Verification items for the finished model (mm, model axes). A direction names the side the tool comes from. Give positions to 0.01 mm unless a question says otherwise; leave off trailing zeros. Order: outer loops, then holes, each group sorted by start corner. A loop starts at its lowest first (then second) coordinate and runs counter-clockwise, first axis right, second up.
from build123d import *

# Parameters (mm, degrees)
BOSS_EXTRUDE1_DEPTH = 6.353
CUT_EXTRUDE1_REACH  = 30.604
SKETCH2_R           = 1.75
SKETCH3_R           = 32.5
CUT_EXTRUDE2_DEPTH  = 9.675
FILLET1_R           = 2.5
CHAMFER1_SIZE       = 10
CHAMFER1_SIZE2      = 1.763269807
CHAMFER2_SIZE       = 10
CHAMFER2_SIZE2      = 1.763269807


with BuildPart() as part:
    # Sketch1 → Boss-Extrude1 (new body)
    with BuildSketch(Plane(origin=(0, 0, 0), x_dir=(0, 0, -1), z_dir=(1, 0, 0))):
        Polygon((0, 19.4375), (-20, 19.4375), (-20, -19.4375), (20, -19.4375), (20, -16.2625), (0, -16.2625), (0, -9.7625), (20, -9.7625), (20, 5.0375), (0, 5.0375), (0, 11.5375), align=None)
    extrude(amount=BOSS_EXTRUDE1_DEPTH)

    # Sketch2 → Cut-Extrude1 (cut, up to next)
    with BuildSketch(Plane(origin=(6.353, 0, 0), x_dir=(0, 0, -1), z_dir=(1, 0, 0)), mode=Mode.PRIVATE) as cut_extrude1_sk1:
        with BuildLine():
            ThreePointArc((-16.45, 5.8875), (-14.7, 7.6375), (-12.95, 5.8875))
            ThreePointArc((-12.95, 5.8875), (-12.455196051, 8.612317472), (-11.033966385, 10.989199346))
            ThreePointArc((-11.033966385, 10.989199346), (-11.199317007, 13.458543221), (-13.668660882, 13.293192599))
            ThreePointArc((-13.668660882, 13.293192599), (-15.731736204, 9.842880202), (-16.45, 5.8875))
        make_face()
    cut_extrude1_tool1 = extrude(cut_extrude1_sk1.sketch, amount=-CUT_EXTRUDE1_REACH, mode=Mode.PRIVATE) & part.part
    # Sketch2 → Cut-Extrude1 (cut, up to next)
    with BuildSketch(Plane(origin=(6.353, 0, 0), x_dir=(0, 0, -1), z_dir=(1, 0, 0)), mode=Mode.PRIVATE) as cut_extrude1_sk2:
        with Locations((-14.7, 5.8875)):
            Circle(SKETCH2_R)
    cut_extrude1_tool2 = extrude(cut_extrude1_sk2.sketch, amount=-CUT_EXTRUDE1_REACH, mode=Mode.PRIVATE) & part.part
    # Sketch2 → Cut-Extrude1 (cut, up to next)
    with BuildSketch(Plane(origin=(6.353, 0, 0), x_dir=(0, 0, -1), z_dir=(1, 0, 0)), mode=Mode.PRIVATE) as cut_extrude1_sk3:
        with Locations((-5.2, 5.8875)):
            Circle(SKETCH2_R)
    cut_extrude1_tool3 = extrude(cut_extrude1_sk3.sketch, amount=-CUT_EXTRUDE1_REACH, mode=Mode.PRIVATE) & part.part
    # Sketch2 → Cut-Extrude1 (cut, up to next)
    with BuildSketch(Plane(origin=(6.353, 0, 0), x_dir=(0, 0, -1), z_dir=(1, 0, 0)), mode=Mode.PRIVATE) as cut_extrude1_sk4:
        Polygon((0, 19.4375), (-20, 19.4375), (-20, 17.296483849), (0, 11.9375), align=None)
    cut_extrude1_tool4 = extrude(cut_extrude1_sk4.sketch, amount=-CUT_EXTRUDE1_REACH, mode=Mode.PRIVATE) & part.part
    add(cut_extrude1_tool1.solids().sort_by_distance((6.353, 10.415401, 13.430466))[0], mode=Mode.SUBTRACT)
    add(cut_extrude1_tool2.solids().sort_by_distance((6.353, 5.8875, 14.7))[0], mode=Mode.SUBTRACT)
    add(cut_extrude1_tool3.solids().sort_by_distance((6.353, 5.8875, 5.2))[0], mode=Mode.SUBTRACT)
    add(cut_extrude1_tool4.solids().sort_by_distance((6.353, 16.779012, 8.147158))[0], mode=Mode.SUBTRACT)

    # Sketch3 → Cut-Extrude2 (cut)
    with BuildSketch(Plane.XZ.offset(19.4375)):
        with Locations((-13, -38.1)):
            Circle(SKETCH3_R)
    extrude(amount=-CUT_EXTRUDE2_DEPTH, mode=Mode.SUBTRACT)

    # Fillet1
    fillet1_edges = [part.edges().sort_by_distance(p)[0] for p in [
        (3.1765, -19.4375, 20),
        (3.1765, 17.296483849, 20),
        (3.1765, 11.9375, 0),
    ]]
    fillet(fillet1_edges, radius=FILLET1_R)

    # Chamfer1
    chamfer1_edges = [part.edges().sort_by_distance(p)[0] for p in [
        (3.1765, 5.0375, -20),
    ]]
    chamfer1_side = [part.faces().sort_by_distance(p)[0] for p in [
        (3.1765, 5.0375, -10),
    ]]
    chamfer(chamfer1_edges, length=CHAMFER1_SIZE, length2=CHAMFER1_SIZE2, reference=chamfer1_side[0])

    # Chamfer2
    chamfer2_edges = [part.edges().sort_by_distance(p)[0] for p in [
        (3.1765, -9.7625, -20),
    ]]
    chamfer2_side = [part.faces().sort_by_distance(p)[0] for p in [
        (3.1765, -9.7625, -10),
    ]]
    chamfer(chamfer2_edges, length=CHAMFER2_SIZE, length2=CHAMFER2_SIZE2, reference=chamfer2_side[0])


solid = part.part
(1) Go/stop test with flat-tipped pins: pin 1 (1.5 mm diameter, centred on x = 2.5, z = -9.5, fed in from +Y); pin 2 (3 mm diameter, centred on x = 3.5, y = -14, fed in from -Z). Record where each tip stops, or that it passes through.
Solved:
pin 1: stops at y = 5.04
pin 2: stops at z = 0
(2) Scan lines: line 1 (Y direction, x = 2.25, z = -1.5); line 2 (Z direction, x = 1, y = -15); line 3 (Y direction, x = 5.5, z = 15). Record each from-to range of solid material in increasing order.
Solved:
line 1: y = -19.44 to -16.26, -9.76 to 5.04
line 2: z = 0 to 20
line 3: y = -19.44 to 4.16, 11.41 to 15.96
(3) Section check C-C, the plane z = 14.7. Enter the section's corners in (x, y), then the cut area to 3 significant figures.
Solved:
outline: (0, -19.44) - (6.35, -19.44) - (6.35, 4.14) - (0, 4.14) - close; (0, 11.91) - (6.35, 11.91) - (6.35, 15.88) - (0, 15.88) - close
area: 175 mm2
(4) Section check B-B, the plane x = 4.25. Enter the section's corners in (y, z).
Solved:
outline: (-19.44, -10.56) - (-16.26, -10.56) - (-16.26, 0) - (-9.76, 0) - (-9.76, -10) - (-8, -20) - (3.27, -20) - (5.04, -10) - (5.04, 0) - (10.02, 0) arc R2.5 ccw to (12.43, 1.85) - (16.45, 16.85) arc R2.5 ccw to (14.04, 20) - (-16.94, 20) arc R2.5 ccw to (-19.44, 17.5) - close; hole circle Ø3.5 at (5.89, 5.2); hole (5.89, 12.95) arc R7.75 cw to (10.99, 11.03) arc R1.75 ccw to (13.29, 13.67) arc R11.25 ccw to (5.89, 16.45) arc R1.75 ccw to start
(5) Set-up check for faces 5 (the cylindrical face through (3.13, 11.52, 0.5)), 6 (the cylindrical face through (3.33, -17.87, -10)), 7 (the cylindrical face through (3.22, 9.9, 15.71)), 8 (the flat face through (3, -13, 0)): record each of +Z, -Z, +X, -X, +Y, -Y from which the full face is reachable in a straight line by a thin tool's end or side.
Solved:
face 5: -Z, +X, -X, +Y
face 6: -Z, -X, -Y
face 7: +X, -X
face 8: -Z, +X, -X
(6) Release check for a two-part mould opening along Z. For faces 1 (the flat face through (3, 5.038, -5)), 2 (the cylindrical face through (3.221, -18.725, 19.248)), 3 (the cylindrical face through (3.221, 8.576, 12.469)), 4 (the flat face through (3.13, -8.87, -15.07)) record: pulls with the +Z half, pulls with the -Z half, needs draft (parallel to the pull), parting line crosses it, or undercut.
Solved:
face 1: needs draft
face 2: pulls with the +Z half
face 3: undercut
face 4: pulls with the -Z half
(7) Section check A-A, the plane z = -1.5. Enter the section's corners in (x, y).
Solved:
outline: (0, -19.44) - (6.35, -19.44) - (6.35, -16.26) - (0, -16.26) - close; (0, -9.76) - (6.35, -9.76) - (6.35, 5.04) - (0, 5.04) - close
(8) Section check D-D, the plane x = 1.75. Enter the section's corners in (y, z), then the cut area to 3 significant figures.
Solved:
outline: (-19.44, -9.14) - (-16.26, -9.14) - (-16.26, 0) - (-9.76, 0) - (-9.76, -10) - (-8, -20) - (3.27, -20) - (5.04, -10) - (5.04, 0) - (10.02, 0) arc R2.5 ccw to (12.43, 1.85) - (16.45, 16.85) arc R2.5 ccw to (14.04, 20) - (-16.94, 20) arc R2.5 ccw to (-19.44, 17.5) - close; hole circle Ø3.5 at (5.89, 5.2); hole (5.89, 12.95) arc R7.75 cw to (10.99, 11.03) arc R1.75 ccw to (13.29, 13.67) arc R11.25 ccw to (5.89, 16.45) arc R1.75 ccw to start
area: 941 mm2
